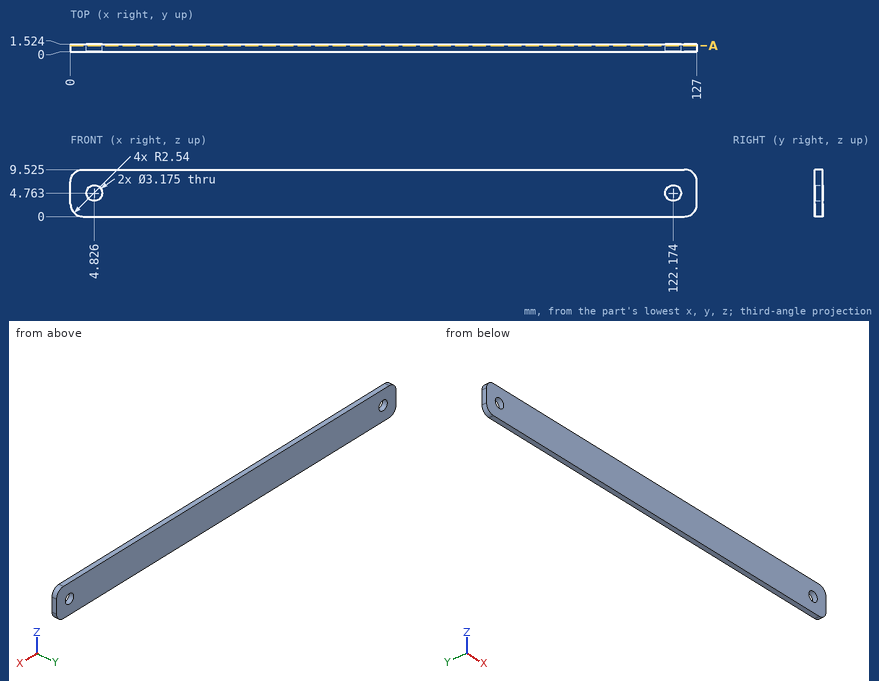
Study the drawing (mm; zero at the part's minimum x, y, z) and answer. Give positions to 0.01 mm unless a question says otherwise; leave off trailing zeros. Order: outer loops, then holes, each group sorted by start corner. A loop starts at its lowest first (then second) coordinate and runs counter-clockwise, first axis right, second up.
1) Given P1, Ø2.5, axis at x = 4.83, z = 4.76, coming from the -Y side, flat-ended and moving along its own axis, determine where the tip first touches the part or whether it passes through.
Reported:
P1: passes through
2) Find section A-A on y = 1.2. Write down the section's boundary in (x, z) (1 decimal), then the cut area to 3 significant figures.
Reported:
outline: (0, 2.5) arc R2.5 ccw to (2.5, 0) - (124.5, 0) arc R2.5 ccw to (127, 2.5) - (127, 7) arc R2.5 ccw to (124.5, 9.5) - (2.5, 9.5) arc R2.5 ccw to (0, 7) - close; hole circle Ø3.2 at (4.8, 4.8); hole circle Ø3.2 at (122.2, 4.8)
area: 1,190 mm2
3) Consider line 1 along X through (y, z) = (0.8, 4.5); line 2 along X through (y, z) = (1.35, 4.75); line 3 along X through (y, z) = (1.45, 8.5). Determine where each line is inside the solid, lowest interval first.
Reported:
line 1: x = 0 to 3.26, 6.39 to 120.61, 123.74 to 127
line 2: x = 0 to 3.24, 6.41 to 120.59, 123.76 to 127
line 3: x = 0.5 to 126.5
